Could you check a few things on this model? Use its own coordinates, in mm. A direction names the side the tool comes from. Give positions to 0.01 mm unless a question says otherwise; leave off trailing zeros. Write each loop counter-clockwise with the first axis right and the second up, starting at its lowest first coordinate (ties: lowest second). Pieces come first, ordered by that corner, then holes. Notation, with made-up numbers: M -40,41.5 L 2,41.5 A25 cw 2,72.5 Z; hole C 74.25,83.25 d7. An arc over 180 degrees is marked long. Answer as a JSON object with one key per item and string values. Group by question number.
```python
from build123d import *

# Parameters (mm, degrees)
SKETCH1_W           = 70
SKETCH1_H           = 109
SKETCH1_R           = 1.6
SKETCH1_W_2         = 15.2
SKETCH1_H_2         = 3.2
BOSS_EXTRUDE1_DEPTH = 3
SKETCH3_W           = 70
SKETCH3_H           = 74
SKETCH3_R           = 1.6
CUT_EXTRUDE1_DEPTH  = 130.576232389
SKETCH4_W           = 12
SKETCH4_H           = 35
SKETCH4_R           = 1.6
BOSS_EXTRUDE2_DEPTH = 3
FILLET3_R           = 10


with BuildPart() as part:
    # Sketch1 → Boss-Extrude1 (new body)
    with BuildSketch(Plane(origin=(0, 0, 0), x_dir=(1, 0, 0), z_dir=(0, 1, 0))):
        with Locations((35, 54.5)):
            Rectangle(SKETCH1_W, SKETCH1_H)
        with Locations(Location((6.8, 6.6, 0), (0, 0, 270))):
            Circle(SKETCH1_R, mode=Mode.SUBTRACT)
        with Locations(Location((63.2, 6.6, 0), (0, 0, 270))):
            Circle(SKETCH1_R, mode=Mode.SUBTRACT)
        with Locations(Location((6.8, 103, 0), (0, 0, 270))):
            Circle(SKETCH1_R, mode=Mode.SUBTRACT)
        with Locations(Location((63.2, 103, 0), (0, 0, 270))):
            Circle(SKETCH1_R, mode=Mode.SUBTRACT)
        with Locations((22.4, 6.6)):
            Rectangle(SKETCH1_W_2, SKETCH1_H_2, mode=Mode.SUBTRACT)
        with Locations((47.6, 6.6)):
            Rectangle(SKETCH1_W_2, SKETCH1_H_2, mode=Mode.SUBTRACT)
    extrude(amount=BOSS_EXTRUDE1_DEPTH)

    # Sketch3 → Cut-Extrude1 (cut, through all)
    with BuildSketch(Plane(origin=(0, 3, 0), x_dir=(1, 0, 0), z_dir=(0, 1, 0))):
        with Locations((35, 72)):
            Rectangle(SKETCH3_W, SKETCH3_H)
        with Locations((6.8, 103)):
            Circle(SKETCH3_R, mode=Mode.SUBTRACT)
        with Locations((63.2, 103)):
            Circle(SKETCH3_R, mode=Mode.SUBTRACT)
    extrude(amount=-CUT_EXTRUDE1_DEPTH, mode=Mode.SUBTRACT)

    # Sketch4 → Boss-Extrude2 (add)
    # profile 1 of 2: a face of its own
    with BuildSketch(Plane(origin=(0, 3, 0), x_dir=(1, 0, 0), z_dir=(0, 1, 0))):
        with Locations((76, 17.5)):
            Rectangle(SKETCH4_W, SKETCH4_H)
        with Locations(Location((76, 27, 0), (0, 0, 270))):
            Circle(SKETCH4_R, mode=Mode.SUBTRACT)
    # profile 2 of 2: a face of its own
    with BuildSketch(Plane(origin=(0, 3, 0), x_dir=(1, 0, 0), z_dir=(0, 1, 0))):
        with Locations((-6, 17.5)):
            Rectangle(SKETCH4_W, SKETCH4_H)
        with Locations(Location((-6, 27, 0), (0, 0, 270))):
            Circle(SKETCH4_R, mode=Mode.SUBTRACT)
    extrude(amount=-BOSS_EXTRUDE2_DEPTH)

    # Fillet3
    fillet3_edges = [part.edges().sort_by_distance(p)[0] for p in [
        (82, 1.5, -35),
        (82, 1.5, 0),
        (-12, 1.5, 0),
        (-12, 1.5, -35),
    ]]
    fillet(fillet3_edges, radius=FILLET3_R)


solid = part.part
```
1) If we section it at B-B, the plane y = 0.45: List the corners of the cut face in (x, z) for me, plus the area to 3 significant figures.
2) If we section it at C-C, the plane z = -27: List the corners of the cut face in (x, y) for me, plus the area to 3 significant figures.
3) If we section it at D-D, the plane z = -6.6: List the corners of the cut face in (x, y) for me.
4) We'd pull the mould along Z, two halves only. Please class faces 3 (the flat face through (40, 1, -7)), 4 (the flat face through (34, 3, -18)), 5 (the cylindrical face through (78.99, 1.48, -2.85)): released by +Z, released by -Z, zero draft, split by the parting line, or undercut.
5) If we section it at A-A, the plane x = 6.8: List the corners of the cut face in (y, z) for me.
6) Please list where these lines run through material, in increasing order: line 1 along X through (y, z) = (1.5, -27); line 2 along X through (y, z) = (0.9, -6.6). Write a range as from..to.
7) For faces 1 (the cylindrical face through (-8.99, 1.48, -2.85)), 2 (the flat face through (47, 1, -8.2)), which set-ups out of +Z, -Z, +X, -X, +Y, -Y let a thin tool reach every point of the face, with its end or its side?
8) I'm going to push flat-ended pins straight in: pin 1 (1 mm diameter, centred on y = 1.5, z = -7, fed in from -X); pin 2 (1.5 mm diameter, centred on y = 2, z = -6.5, fed in from -X); pin 3 (0.9 mm diameter, centred on y = 1.5, z = -7, fed in from +X). Where does each tip first touch, or does it pass through?
Taken from the geometry:
{
 "1": {"outline": "M -12,-25 A10 ccw -2,-35 L 72,-35 A10 ccw 82,-25 L 82,-10 A10 ccw 72,0 L -2,0 A10 ccw -12,-10 Z; hole C -6,-27 d3.2; hole C 6.8,-6.6 d3.2; hole M 14.8,-8.2 L 30,-8.2 L 30,-5 L 14.8,-5 Z; hole M 40,-8.2 L 55.2,-8.2 L 55.2,-5 L 40,-5 Z; hole C 63.2,-6.6 d3.2; hole C 76,-27 d3.2", "area": "3,070 mm²"},
 "2": {"outline": "M -11.8,0 L -7.6,0 L -7.6,3 L -11.8,3 Z; M -4.4,0 L 74.4,0 L 74.4,3 L -4.4,3 Z; M 77.6,0 L 81.8,0 L 81.8,3 L 77.6,3 Z", "area": "262 mm²"},
 "3": {"outline": "M -11.4,0 L 5.2,0 L 5.2,3 L -11.4,3 Z; M 8.4,0 L 14.8,0 L 14.8,3 L 8.4,3 Z; M 30,0 L 40,0 L 40,3 L 30,3 Z; M 55.2,0 L 61.6,0 L 61.6,3 L 55.2,3 Z; M 64.8,0 L 81.4,0 L 81.4,3 L 64.8,3 Z"},
 "4": {"face 3": "undercut", "face 4": "zero draft", "face 5": "released by +Z"},
 "5": {"outline": "M 0,-35 L 3,-35 L 3,-8.2 L 0,-8.2 Z; M 0,-5 L 3,-5 L 3,0 L 0,0 Z"},
 "6": {"line 1": "-11.8..-7.6, -4.4..74.4, 77.6..81.8", "line 2": "-11.4..5.2, 8.4..14.8, 30..40, 55.2..61.6, 64.8..81.4"},
 "7": {"face 1": "+Z, -X, +Y, -Y", "face 2": "+Y, -Y"},
 "8": {"pin 1": "x = -11.68", "pin 2": "x = -11.61", "pin 3": "x = 81.67"}
}
